Read the model definition and answer for the solid it produces. Units are mm, in the model's axes. Face numbers are marked on the shaded views. A direction names the side the tool comes from. Coordinates: 2 decimals unless noted, no trailing zeros. Write each loop counter-clockwise with the first axis right and the second up, starting at its lowest first coordinate (ties: lowest second). Pieces come first, ordered by that corner, then holes. Notation, with made-up numbers: (84.25, 16.25) - (99.25, 16.25) arc R26 ccw to (99.25, 51.25) - close; hole circle Ø10 at (6, 55). An arc over 180 degrees is marked (long way). Use a Markdown table: item, result.
from build123d import *

# Parameters (mm, degrees)
SKETCH_1_W           = 14.8
SKETCH_1_H           = 13
EXTRUDE_1_DEPTH      = 14.2
SKETCH_2_R           = 6.4
EXTRUDE_2_DEPTH      = 8.6
SKETCH_3_R           = 5.5
SKETCH_3_R_2         = 5
EXTRUDE_3_DEPTH      = 12.1
EXTRUDE_4_DEPTH      = 6
EXTRUDE_4_DEPTH_BACK = 6
SKETCH_4_W           = 1
SKETCH_4_H           = 1
SKETCH_7_R           = 0.95
SKETCH_7_R_2         = 0.4
EXTRUDE_5_DEPTH      = 3.3


with BuildPart() as part:
    # Эскиз1 → Бобышка-Вытянуть1 (new body)
    with BuildSketch(Plane.XY):
        Rectangle(SKETCH_1_W, SKETCH_1_H)
    extrude(amount=-EXTRUDE_1_DEPTH)

    # Эскиз2 → Бобышка-Вытянуть2 (add)
    with BuildSketch(Plane(origin=(0, 0, -14.2), x_dir=(-1, 0, 0), z_dir=(0, 0, -1))):
        with Locations(Location((0, 0, 0), (0, 0, 180))):
            Circle(SKETCH_2_R)
    extrude(amount=EXTRUDE_2_DEPTH)

    # Эскиз3 → Бобышка-Вытянуть3 (add)
    with BuildSketch(Plane(origin=(0, 0, -22.8), x_dir=(-1, 0, 0), z_dir=(0, 0, -1))):
        Circle(SKETCH_3_R)
        Circle(SKETCH_3_R_2, mode=Mode.SUBTRACT)
    extrude(amount=EXTRUDE_3_DEPTH)

    # Эскиз4 → Бобышка-Вытянуть4 (add, two sides: drawn at the far end of the back side and taken through both)
    with BuildSketch(Plane(origin=(0, 0, 0), x_dir=(0, 0, -1), z_dir=(1, 0, 0)).offset(-EXTRUDE_4_DEPTH_BACK)):
        with Locations((31, 0)):
            Rectangle(SKETCH_4_W, SKETCH_4_H)
    extrude(amount=EXTRUDE_4_DEPTH + EXTRUDE_4_DEPTH_BACK)

    # Эскиз7 → Бобышка-Вытянуть5 (add)
    with BuildSketch(Plane.XZ.offset(6.5)):
        with Locations(Location((5.08, -6.8, 0), (0, 0, 270))):
            Circle(SKETCH_7_R)
        with Locations(Location((-5.08, -6.8, 0), (0, 0, 270))):
            Circle(SKETCH_7_R)
        with Locations(Location((0, -1.72, 0), (0, 0, 270))):
            Circle(SKETCH_7_R_2)
        with Locations(Location((-2.54, -1.72, 0), (0, 0, 270))):
            Circle(SKETCH_7_R_2)
    extrude(amount=EXTRUDE_5_DEPTH)


solid = part.part
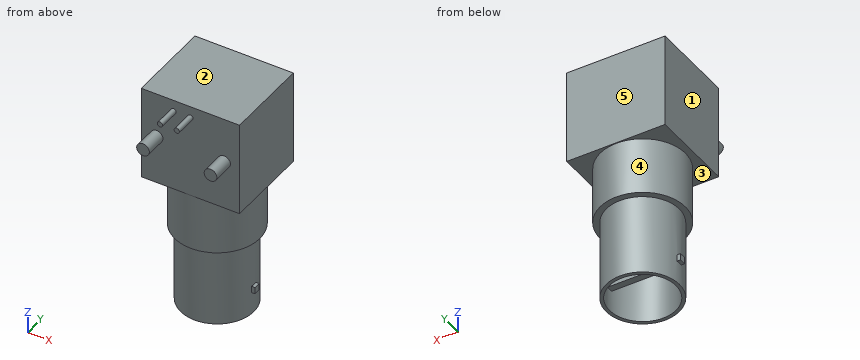
(1) A cutting plane is placed at B-B, the plane y = 0. Write down the section's boundary in (x, z).
Report:
| item | result |
|---|---|
| outline | (-7.4, -14.2) - (-6.4, -14.2) - (-6.4, -22.8) - (-5.5, -22.8) - (-5.5, -30.5) - (-6, -30.5) - (-6, -31.5) - (-5.5, -31.5) - (-5.5, -34.9) - (-5, -34.9) - (-5, -31.5) - (5, -31.5) - (5, -34.9) - (5.5, -34.9) - (5.5, -31.5) - (6, -31.5) - (6, -30.5) - (5.5, -30.5) - (5.5, -22.8) - (6.4, -22.8) - (6.4, -14.2) - (7.4, -14.2) - (7.4, 0) - (-7.4, 0) - close; hole (-5, -30.5) - (5, -30.5) - (5, -22.8) - (-5, -22.8) - close |
(2) Straight lines are drawn through the part: L1, parallel to X at y = 0, z = -26.5; L2, parallel to Z at x = -5.5, y = -2.5. For each, find the intervals that lie inside material, in ascending order.
Report:
| item | result |
|---|---|
| L1 | x = -5.5 to -5, 5 to 5.5 |
| L2 | z = -22.8 to 0 |
(3) For the marked faces 4 and 5, determine the directions among +Z, -Z, +X, -X, +Y, -Y from which every point of the face is accessible in a straight line to the end or side of a thin tool.
Report:
| item | result |
|---|---|
| face 4 | -Z |
| face 5 | +Z, -Z, +X, -X, +Y |
(4) A cutting plane is placed at A-A, the plane x = -1. Write down the section's boundary in (y, z).
Report:
| item | result |
|---|---|
| outline | (-6.5, -14.2) - (-6.32, -14.2) - (-6.32, -22.8) - (-5.41, -22.8) - (-5.41, -34.9) - (-4.9, -34.9) - (-4.9, -22.8) - (4.9, -22.8) - (4.9, -34.9) - (5.41, -34.9) - (5.41, -22.8) - (6.32, -22.8) - (6.32, -14.2) - (6.5, -14.2) - (6.5, 0) - (-6.5, 0) - close; (-0.5, -31.5) - (0.5, -31.5) - (0.5, -30.5) - (-0.5, -30.5) - close |
(5) A cutting plane is placed at D-D, the plane y = -7.25. Write down the section's boundary in (x, z).
Report:
| item | result |
|---|---|
| outline | circle Ø1.9 at (-5.08, -6.8); circle Ø0.8 at (-2.54, -1.72); circle Ø0.8 at (0, -1.72); circle Ø1.9 at (5.08, -6.8) |
(6) The mould has two halves that part along Z. Classify the marked faces 1, 2 and 3: pulls with the +Z half, pulls with the -Z half, needs draft (parallel to the pull), parting line crosses it, or undercut.
Report:
| item | result |
|---|---|
| face 1 | needs draft |
| face 2 | pulls with the +Z half |
| face 3 | pulls with the -Z half |
(7) Each of these flat-tipped pins is pushed along its axis until it touches: P1, Ø4, axis at x = 4.5, y = -4, coming from the +Z side; P2, Ø1.5, axis at x = 0, y = -2.5, coming from the -Z side; P3, Ø2, axis at x = 4.5, z = -16.5, coming from the -Y side; P4, Ø8, axis at y = -6.5, z = -22, coming from the -X side. Where does it stop, or does it pass through?
Report:
| item | result |
|---|---|
| P1 | stops at z = 0 |
| P2 | stops at z = -22.8 |
| P3 | stops at y = -5.36 |
| P4 | stops at x = -5.89 |
(8) A cutting plane is placed at C-C, the plane z = -1.72. Write down the section's boundary in (x, y).
Report:
| item | result |
|---|---|
| outline | (-7.4, -6.5) - (-2.94, -6.5) - (-2.94, -9.8) - (-2.14, -9.8) - (-2.14, -6.5) - (-0.4, -6.5) - (-0.4, -9.8) - (0.4, -9.8) - (0.4, -6.5) - (7.4, -6.5) - (7.4, 6.5) - (-7.4, 6.5) - close |
